from build123d import *

# Parameters (mm, degrees)
F0_W     = 54
F0_H     = 84
F1_DEPTH = 1.2
F0_W_2   = 1.2
F2_DEPTH = 55
F3_W     = 10
F3_H     = 10
F4_DEPTH = 25


with BuildPart() as f1:
    # F0 (on Top) → F1 (new body)
    with BuildSketch(Plane.XY):
        Rectangle(F0_W, F0_H)
    extrude(amount=F1_DEPTH)

    # F0 (on Top) → F2 (join)
    with BuildSketch(Plane.XY):
        with Locations((-27.6, 0)):
            Rectangle(F0_W_2, F0_H)
        with Locations((27.6, 0)):
            Rectangle(F0_W_2, F0_H)
    extrude(amount=F2_DEPTH)

    # F3 (on face) → F4 (cut)
    with BuildSketch(Plane.YZ.offset(28.2)):
        with Locations((-25, 50)):
            Rectangle(F3_W, F3_H)
        with Locations((25, 50)):
            Rectangle(F3_W, F3_H)
    extrude(amount=-F4_DEPTH, mode=Mode.SUBTRACT)


solid = f1.part
Geometry check sheet. Reference: the model listing, model coordinates, mm. A direction names the side the tool comes from. Coordinates: 2 decimals unless noted, no trailing zeros. Loops run counter-clockwise (first coordinate to the right, second up) from the corner with the lowest first, then second, coordinate; pieces in that order, holes last. Notation, with made-up numbers: (51.5, 55) - (82.5, 55) arc R20 cw to (82.5, 90) - close; hole circle Ø5 at (0, 82). An arc over 180 degrees is marked (long way). Use one line per item in the form item = value. Start each with the question number.
Item 1: Section check A-A, the plane z = 47. Enter the section's corners in (x, y).
Item 2: Gauge pin test, flat ends, axial feed: pin 1 (1 mm diameter, centred on x = -5.5, y = -5.5, fed in from +Z); pin 2 (1.3 mm diameter, centred on x = 27.5, y = -25.5, fed in from +Z). Record the tip position at first contact, or that the pin passes through.
Item 3: Mould release check, pull along X, two halves, no side actions. Record for faces 3 (the face through (0, 42, 1)), 4 (the face through (28.2, -1, 27)), 5 (the face through (-28.2, -1, 27)), 6 (the face through (-27, -1, 28)): +X half, -X half, draft (parallel to the pull), parting line (faces both ways), or undercut.
Item 4: Section check C-C, the plane y = 27. Enter the section's corners in (x, z).
Item 5: Section check D-D, the plane x = -13. Enter the section's corners in (y, z).
Item 6: Section check B-B, the plane y = -11. Enter the section's corners in (x, z).
Item 7: Thickness scan on probe 1 along X at (y, z) = (3, 7); probe 2 along Z at (x, y) = (20, 4.5). Record the ranges inside material, lowest first.
Item 8: Tool access check on faces 1 (the face through (0, 1, 1.2)), 2 (the face through (0, 1, 0)). Record the directions out of +Z, -Z, +X, -X, +Y, -Y that give a thin tool (end or side, any length) a straight path to the whole face; none if there is none.
Computed:
q1.outline = (-28.2, -42) - (-27, -42) - (-27, 42) - (-28.2, 42) - close; (27, -42) - (28.2, -42) - (28.2, -30) - (27, -30) - close; (27, -20) - (28.2, -20) - (28.2, 20) - (27, 20) - close; (27, 30) - (28.2, 30) - (28.2, 42) - (27, 42) - close
q2.pin_1 = 1.2
q2.pin_2 = 45
q3.face_3 = draft
q3.face_4 = +X half
q3.face_5 = -X half
q3.face_6 = undercut
q4.outline = (-28.2, 0) - (28.2, 0) - (28.2, 45) - (27, 45) - (27, 1.2) - (-27, 1.2) - (-27, 55) - (-28.2, 55) - close
q5.outline = (-42, 0) - (42, 0) - (42, 1.2) - (-42, 1.2) - close
q6.outline = (-28.2, 0) - (28.2, 0) - (28.2, 55) - (27, 55) - (27, 1.2) - (-27, 1.2) - (-27, 55) - (-28.2, 55) - close
q7.probe_1 = -28.2 to -27, 27 to 28.2
q7.probe_2 = 0 to 1.2
q8.face_1 = +Z, +Y, -Y
q8.face_2 = -Z, +X, -X, +Y, -Y
